Can you work these out from the model? Positions are in its coordinate system, mm. Give positions to 0.01 mm unless a question says otherwise; leave off trailing zeros. Loops run counter-clockwise (first coordinate to the right, second up) from the corner with the lowest first, then second, coordinate; pieces in that order, holes last. Notation, with made-up numbers: M -29,45.25 L 29,45.25 A31 ccw 29,71.25 Z; hole C 47,72.5 d3. An arc over 180 degrees is marked long. Put each result on its own line as item: value. Start each with the question number.
1) Imagine slicing it at B-B (x = 15.5). Write out the boundary of the cut face in (y, z).
2) Please list where these lines run through material, in increasing order: line 1 along Z through (x, y) = (-8, 21); line 2 along X through (y, z) = (64, -14.2); line 3 along Y through (x, z) = (-11.5, -14.8). Write a range as from..to.
3) Imagine slicing it at A-A (y = 22.5). Write out the boundary of the cut face in (x, z), then the cut area to 3 significant figures.
4) For P1, Ø14, axis at x = -5.5, y = 24.5, coming from the -Z side; P2, Ø1, axis at y = 35, z = -14, coming from the -X side; P3, Ø0.8, axis at y = 72.5, z = -16, coming from the +X side, each with a flat end and sliding along its axis, tell me the tip position at first contact or that it passes through.
5) Imagine slicing it at D-D (x = 3). Write out the boundary of the cut face in (y, z), then the cut area to 3 significant figures.
6) Imagine slicing it at C-C (z = -14.2). Write out the boundary of the cut face in (x, y).
from build123d import *

# Parameters (mm, degrees)
BOSS_EXTRUDE2_DEPTH = 75.66
SKETCH2_W           = 2
SKETCH2_H           = 2
CUT_EXTRUDE2_DEPTH  = 69
FILLET1_R           = 2
BOSS_EXTRUDE5_DEPTH = 1


with BuildPart() as part:
    # Sketch1 → Boss-Extrude2 (new body)
    with BuildSketch(Plane(origin=(0, 0, 0), x_dir=(1, 0, 0), z_dir=(0, 1, 0))):
        Polygon((-19.20717284, 15.283675177), (27.59282716, 15.283675177), (27.59282716, 13.283675177), (29.59282716, 13.283675177), (29.59282716, 11.283675177), (-21.20717284, 11.283675177), (-21.20717284, 13.283675177), (-19.20717284, 13.283675177), align=None)
    extrude(amount=BOSS_EXTRUDE2_DEPTH)

    # Sketch2 → Cut-Extrude2 (cut)
    with BuildSketch(Plane(origin=(27.59282716, 0, 0), x_dir=(0, 0, -1), z_dir=(1, 0, 0))):
        with Locations((14.283675177, 1)):
            Rectangle(SKETCH2_W, SKETCH2_H)
    extrude(amount=-CUT_EXTRUDE2_DEPTH, mode=Mode.SUBTRACT)

    # Fillet1
    fillet1_edges = [part.edges().sort_by_distance(p)[0] for p in [
        (4.19282716, 75.66, -15.283675177),
    ]]
    fillet(fillet1_edges, radius=FILLET1_R)

    # Sketch3 → Boss-Extrude5 (add)
    with BuildSketch(Plane(origin=(0, 0, -15.283675177), x_dir=(-1, 0, 0), z_dir=(0, 0, -1))):
        Polygon((2.614345679, 73.441300995), (-8.385654321, 73.441300995), (-9.385654321, 73.441300995), (-9.385654321, 71.441300995), (-8.385654321, 71.441300995), (2.614345679, 71.441300995), align=None)
    extrude(amount=BOSS_EXTRUDE5_DEPTH)


solid = part.part
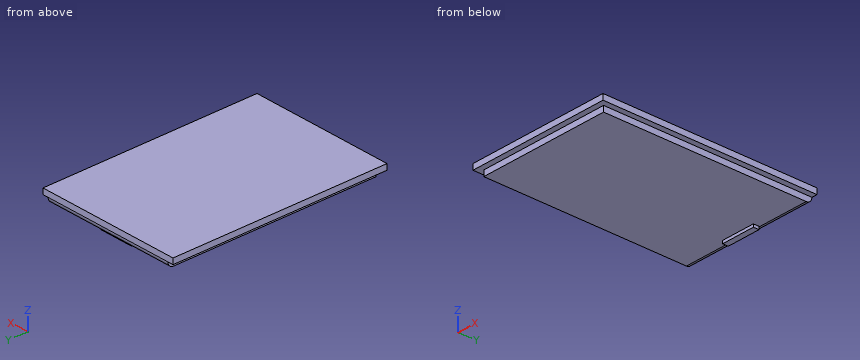
Recorded:
1. outline: M 0,-13.28 L 2,-13.28 L 2,-15.28 L 73.66,-15.28 A2 ccw 75.66,-13.28 L 75.66,-11.28 L 0,-11.28 Z
2. line 1: -15.28..-11.28
2. line 2: -19.21..27.59
2. line 3: 2..74.96
3. outline: M -21.21,-13.28 L -19.21,-13.28 L -19.21,-15.28 L 27.59,-15.28 L 27.59,-13.28 L 29.59,-13.28 L 29.59,-11.28 L -21.21,-11.28 Z
3. area: 195 mm²
4. P1: z = -15.28
4. P2: x = -19.21
4. P3: x = 9.39
5. outline: M 0,-13.28 L 2,-13.28 L 2,-15.28 L 71.44,-15.28 L 71.44,-16.28 L 73.44,-16.28 L 73.44,-15.28 L 73.66,-15.28 A2 ccw 75.66,-13.28 L 75.66,-11.28 L 0,-11.28 Z
5. area: 300 mm²
6. outline: M -19.21,2 L 27.59,2 L 27.59,75.44 L -19.21,75.44 Z
